Can you work these out from the model? Positions are in its coordinate system, mm. A direction names the side the tool comes from. Give positions to 0.01 mm unless a question says otherwise; leave off trailing zeros. Write each loop counter-clockwise with the first axis right and the second up, starting at its lowest first coordinate (ties: lowest second). Pieces come first, ordered by that corner, then holes.
from build123d import *

# Parameters (mm, degrees)
SKETCH_3_W      = 35
SKETCH_3_H      = 40
EXTRUDE_1_DEPTH = 5
EXTRUDE_2_DEPTH = 3.5
SKETCH_5_W      = 35
SKETCH_5_H      = 40
EXTRUDE_3_DEPTH = 5
SKETCH_6_W      = 2
SKETCH_6_H      = 1.5
SKETCH_6_W_2    = 1.5
SKETCH_6_H_2    = 2
EXTRUDE_4_DEPTH = 3.1


with BuildPart() as part:
    # 草图3 → 凸台-拉伸1 (new body)
    with BuildSketch(Plane.XY):
        with Locations((0, 20)):
            Rectangle(SKETCH_3_W, SKETCH_3_H)
        with BuildLine():
            Line((4.6, 26.8), (4.6, 13.6))
            ThreePointArc((4.6, 13.6), (0, 9), (-4.6, 13.6))
            Line((-4.6, 13.6), (-4.6, 26.8))
            ThreePointArc((-4.6, 26.8), (0, 31.4), (4.6, 26.8))
        make_face(mode=Mode.SUBTRACT)
    extrude(amount=EXTRUDE_1_DEPTH)

    # 草图4 → 凸台-拉伸2 (add)
    with BuildSketch(Plane.ZY.offset(17.5)):
        Polygon((5, 40), (8.5, 40), (8.5, 31.8), (31.8, 8.5), (40, 8.5), (40, 0), (5, 0), align=None)
    extrude_2 = extrude(amount=-EXTRUDE_2_DEPTH)

    # 镜向1: 凸台-拉伸2 across plane
    add(extrude_2.mirror(Plane(origin=(0, 0, 0), x_dir=(0, 0, 1), z_dir=(1, 0, 0))))

    # 草图5 → 凸台-拉伸3 (add)
    with BuildSketch(Plane.XZ):
        with Locations((0, 20)):
            Rectangle(SKETCH_5_W, SKETCH_5_H)
        with BuildLine():
            Line((4.6, 26.8), (4.6, 13.6))
            ThreePointArc((4.6, 13.6), (0, 9), (-4.6, 13.6))
            Line((-4.6, 13.6), (-4.6, 26.8))
            ThreePointArc((-4.6, 26.8), (0, 31.4), (4.6, 26.8))
        make_face(mode=Mode.SUBTRACT)
    extrude(amount=-EXTRUDE_3_DEPTH)

    # 草图6 → 凸台-拉伸4 (add, symmetric)
    with BuildSketch(Plane(origin=(0, 0, 0), x_dir=(0, 0, -1), z_dir=(1, 0, 0))):
        with Locations((-35, -0.75)):
            Rectangle(SKETCH_6_W, SKETCH_6_H)
        with Locations((-5, -0.75)):
            Rectangle(SKETCH_6_W, SKETCH_6_H)
        with Locations((0.75, 5)):
            Rectangle(SKETCH_6_W_2, SKETCH_6_H_2)
        with Locations((0.75, 35)):
            Rectangle(SKETCH_6_W_2, SKETCH_6_H_2)
    extrude(amount=EXTRUDE_4_DEPTH, both=True)


solid = part.part
(1) Imagine slicing it at B-B, the plane y = 17.5. Write out the boundary of the cut face in (x, z), plus the area to 3 significant figures.
Returned:
outline: (-17.5, 0) - (-4.6, 0) - (-4.6, 5) - (-14, 5) - (-14, 22.8) - (-17.5, 22.8) - close; (4.6, 0) - (17.5, 0) - (17.5, 22.8) - (14, 22.8) - (14, 5) - (4.6, 5) - close
area: 254 mm2
(2) Imagine slicing it at A-A, the plane x = 0. Give the number of separate pieces and of enclosed holes in the cut face, plus the area to 3 significant figures.
Returned:
separate pieces: 3
enclosed holes: 0
area: 163 mm2
(3) Will these pins go through, and if not, where does the flat tip stop? P1, Ø1.2, axis at y = 35.5, z = -1, coming from the -X side; P2, Ø5, axis at x = 1, y = 12, coming from the +Z side; P3, Ø8, axis at x = -11.5, z = 24.5, coming from the -Y side; P4, Ø1.6, axis at x = -1, z = -1, coming from the -Y side.
Returned:
P1: stops at x = -3.1
P2: passes through
P3: stops at y = 0
P4: stops at y = 4
(4) If I drill on L1, parallel to X at y = 18, z = 12; L2, parallel to Y at x = -13.5, z = 8.5, over which ranges is the centre line in solid material (lowest first)?
Returned:
L1: x = -17.5 to -14, 14 to 17.5
L2: y = 0 to 5
(5) Imagine slicing it at D-D, the plane y = 2. Write out the boundary of the cut face in (x, z), plus the area to 3 significant figures.
Returned:
outline: (-17.5, 0) - (17.5, 0) - (17.5, 40) - (-17.5, 40) - close; hole (-4.6, 13.6) arc R4.6 ccw to (4.6, 13.6) - (4.6, 26.8) arc R4.6 ccw to (-4.6, 26.8) - close
area: 1,210 mm2
(6) Imagine slicing it at C-C, the plane z = 18.5. Write out the boundary of the cut face in (x, y), plus the area to 3 significant figures.
Returned:
outline: (-17.5, 0) - (-4.6, 0) - (-4.6, 5) - (-14, 5) - (-14, 21.8) - (-17.5, 21.8) - close; (4.6, 0) - (17.5, 0) - (17.5, 21.8) - (14, 21.8) - (14, 5) - (4.6, 5) - close
area: 247 mm2
(7) If we mould it in two halves opening along X, with no side actions, what happens to faces 6 (the face through (-3.1, -1, 35)), 7 (the face through (0, 40, 3)), 8 (the face through (6, 5, 23))? For each: +X half, -X half, draft (parallel to the pull), parting line (faces both ways), or undercut.
Returned:
face 6: -X half
face 7: draft
face 8: undercut
(8) For faces 1 (the face through (0, -1, 4)), 2 (the face through (0, 9, 2)), 3 (the face through (0, 36, -1)), 4 (the face through (0, -1, 36)), 5 (the face through (0, 6, -1)), which set-ups out of +Z, -Z, +X, -X, +Y, -Y let a thin tool reach every point of the face, with its end or its side?
Returned:
face 1: -Z, +X, -X, -Y
face 2: +Z, -Z
face 3: -Z, +X, -X, +Y
face 4: +Z, +X, -X, -Y
face 5: -Z, +X, -X
